Read the model definition and answer for the solid it produces. Units are mm, in the model's axes. A direction names the side the tool comes from. Give positions to 0.01 mm unless a question says otherwise; leave off trailing zeros. Write each loop counter-clockwise with the first axis right and the second up, starting at its lowest first coordinate (ties: lowest second). Pieces come first, ordered by that corner, then holes.
```python
from build123d import *

# Parameters (mm, degrees)
F0_R        = 2
F0_R_2      = 4.682431568
F1_DEPTH    = 10
F0_R_3      = 3.1
F0_R_4      = 1.575
F2_DEPTH    = 15
F1_FACE_R   = 2
F1_FACE_R_2 = 4.682431568
F3_DEPTH    = 3
F5_DEPTH    = 6
F6_R        = 1


with BuildPart() as f1:
    # F0 (on Top) → F1 (new body)
    with BuildSketch(Plane.XY):
        with BuildLine():
            ThreePointArc((9.3908199855, -8.25), (11.6969066385, -4.4082167699), (12.5, 0))
            ThreePointArc((12.5, 0), (-4.4082167699, 11.6969066385), (-9.3908199855, -8.25))
            Line((-9.3908199855, -8.25), (9.3908199855, -8.25))
        make_face()
        with Locations((-7.3612159322, -4.25)):
            Circle(F0_R, mode=Mode.SUBTRACT)
        with Locations((7.3612159322, -4.25)):
            Circle(F0_R, mode=Mode.SUBTRACT)
        Circle(F0_R_2, mode=Mode.SUBTRACT)
        with Locations((0, 8.5)):
            Circle(F0_R, mode=Mode.SUBTRACT)
    extrude(amount=F1_DEPTH)

    # F0 (on Top) → F2 (join)
    with BuildSketch(Plane.XY):
        Circle(F0_R_2)
        Circle(F0_R_3, mode=Mode.SUBTRACT)
        Circle(F0_R_3)
        Circle(F0_R_4, mode=Mode.SUBTRACT)
    extrude(amount=F2_DEPTH)

    # F1_face (on face) + F0 (on Top) → F3 (cut)
    with BuildSketch(Plane(origin=(0, 1.6783251384, 10), x_dir=(1, 0, 0), z_dir=(0, 0, 1))):
        with BuildLine():
            ThreePointArc((9.3908199855, -9.9283251384), (0, 10.8216748616), (-9.3908199855, -9.9283251384))
            Line((-9.3908199855, -9.9283251384), (9.3908199855, -9.9283251384))
        make_face()
        with Locations((-7.3612159322, -5.9283251384)):
            Circle(F1_FACE_R, mode=Mode.SUBTRACT)
        with Locations((7.3612159322, -5.9283251384)):
            Circle(F1_FACE_R, mode=Mode.SUBTRACT)
        with Locations((0, -1.6783251384)):
            Circle(F1_FACE_R_2, mode=Mode.SUBTRACT)
        with Locations((0, 6.8216748616)):
            Circle(F1_FACE_R, mode=Mode.SUBTRACT)
    with BuildSketch(Plane.XY):
        Circle(F0_R_3)
        Circle(F0_R_4, mode=Mode.SUBTRACT)
    extrude(amount=F3_DEPTH, mode=Mode.SUBTRACT)

    # F4 (on Top) → F5 (cut)
    with BuildSketch(Plane.XY):
        Polygon((2.7, -1.5588457268), (2.7, 1.5588457268), (0, 3.1176914536), (-2.7, 1.5588457268), (-2.7, -1.5588457268), (0, -3.1176914536), align=None)
    extrude(amount=F5_DEPTH, mode=Mode.SUBTRACT)

    # F6
    f6_edges = [f1.edges().sort_by_distance(p)[0] for p in [
        (-1.575, 0, 15),
        (-4.682432, 0, 15),
        (-4.682432, 0, 10),
        (0, 12.5, 10),
        (0, -8.25, 10),
        (0, 12.5, 0),
        (0, -8.25, 0),
        (9.39082, -8.25, 5),
        (-9.39082, -8.25, 5),
    ]]
    fillet(f6_edges, radius=F6_R)


solid = f1.part
```
Item 1: Determine the mould class of faces 1 (the cylindrical face through (4.466, 1.406, 12.479)), 2 (the flat face through (0, -8.25, 5)), 3 (the cylindrical face through (1.531, -2.696, 1.479)) for opening direction Y: pulls with the +Y half, pulls with the -Y half, needs draft (parallel to the pull), parting line crosses it, or undercut.
Result set:
face 1: parting line crosses it
face 2: pulls with the -Y half
face 3: undercut
Item 2: Section A-A (z = 12.5) is taken. Write down the section's boundary in (x, y) (3 decimals), and give its area (3 significant figures).
Result set:
outline: circle Ø9.365 at (0, 0); hole circle Ø3.15 at (0, 0)
area: 61.1 mm2
Item 3: Each of these flat-tipped pins is pushed along its axis until it touches: pin 1 Ø5 at (y, z) = (5, 9) entering from +X; pin 2 Ø3 at (x, y) = (-7, 10) entering from +Z; pin 3 Ø2.5 at (x, y) = (0.5, 1) entering from -Z; pin 4 Ø3.5 at (x, y) = (7.36, -4.25) entering from +Z. Where does it stop, or does it pass through?
Result set:
pin 1: stops at x = 12.25
pin 2: stops at z = 10
pin 3: stops at z = 6
pin 4: passes through
Item 4: Section B-B (y = -4.25) is taken. Give the number of separate pieces and of enclosed holes in the cut face, and give its area (3 significant figures).
Result set:
separate pieces: 3
enclosed holes: 0
area: 173 mm2
Item 5: Find the intervals of material crossed by line 1 along Y through (x, z) = (0, 8) (3 decimals); line 2 along Z through (x, y) = (4.5, 9.75); line 3 along Y through (x, z) = (-1, 5.5), in increasing order.
Result set:
line 1: y = -8.25 to -1.575, 1.575 to 6.5, 10.5 to 12.5
line 2: z = 0 to 10
line 3: y = -8.25 to -2.54, 2.54 to 6.77, 10.23 to 12.46
Item 6: Which of the six approach directions +Z, -Z, +X, -X, +Y, -Y give full straight-line access (tool end or side, diameter ignored) to faces 4 (the flat face through (-1.5, -2.5, 3)), 5 (the cylindrical face through (6.928, -6.202, 4.93))?
Result set:
face 4: -Z
face 5: +Z, -Z
